The listing builds one solid part. Answer for the finished solid, in the listing's coordinates (mm). A direction names the side the tool comes from. Coordinates: 2 decimals unless noted, no trailing zeros. Write each loop counter-clockwise with the first axis right and the second up, starting at its lowest first coordinate (ties: lowest second). Pieces come first, ordered by that corner, then holes.
from build123d import *

# Parameters (mm, degrees)
SKETCH1_R      = 2.54
EXTRUDE1_DEPTH = 38.1
CHAMFER1_SIZE  = 0.508
EXTRUDE7_DEPTH = 26.4


with BuildPart() as part:
    # Sketch1 → Extrude1 (new body, symmetric)
    with BuildSketch(Plane.XY):
        Circle(SKETCH1_R)
    extrude(amount=EXTRUDE1_DEPTH, both=True)

    # Chamfer1
    chamfer1_edges = [part.edges().sort_by_distance(p)[0] for p in [
        (-2.54, 0, -38.1),
        (-2.54, 0, 38.1),
    ]]
    chamfer(chamfer1_edges, length=CHAMFER1_SIZE)

    # Sketch13 → Extrude7 (cut, through all)
    with BuildSketch(Plane.XY.offset(12.7)):
        with BuildLine():
            Line((-1.27, 2.199704526), (1.27, 2.199704526))
            ThreePointArc((1.27, 2.199704526), (0, 2.54), (-1.27, 2.199704526))
        make_face()
    extrude(amount=EXTRUDE7_DEPTH, mode=Mode.SUBTRACT)


solid = part.part
Q1. Find the intervals of material crossed by probe 1 along X at (y, z) = (2.2, -15); probe 2 along X at (y, z) = (0.1, -16.5), in increasing order.
Answers below:
probe 1: x = -1.27 to 1.27
probe 2: x = -2.54 to 2.54
Q2. The part is cut by section B-B, the plane z = -9. Write down the section's boundary in (x, y).
Answers below:
outline: circle Ø5.08 at (0, 0)
Q3. The part is cut by section A-A, the plane x = 0. Write down the section's boundary in (y, z), then the cut area to 3 significant figures.
Answers below:
outline: (-2.54, -37.59) - (-2.03, -38.1) - (2.03, -38.1) - (2.54, -37.59) - (2.54, 12.7) - (2.2, 12.7) - (2.2, 37.93) - (2.03, 38.1) - (-2.03, 38.1) - (-2.54, 37.59) - close
area: 378 mm2
Q4. Given pin 1 (3 mm diameter, centred on x = -0.5, z = 24.5, fed in from +Y), flat-ended and moving along its own axis, determine where the tip first touches the part or whether it passes through.
Answers below:
pin 1: stops at y = 2.2
Q5. Which of the six approach directions +Z, -Z, +X, -X, +Y, -Y give full straight-line access (tool end or side, diameter ignored) to faces 1 (the face through (0, 2.2, 25)), 2 (the face through (-0.55, -2.48, 0.53))?
Answers below:
face 1: +Z, +X, -X, +Y
face 2: +Z, -Z
Q6. The part is cut by section C-C, the plane z = 17. Write down the section's boundary in (x, y).
Answers below:
outline: (-1.27, 2.2) arc R2.54 ccw (long way) to (1.27, 2.2) - close
